from build123d import *

# Parameters (mm, degrees)
BOSS_EXTRU_1_DEPTH = 6


with BuildPart() as part:
    # Esquisse1 → Boss.-Extru.1 (new body)
    with BuildSketch(Plane.XY):
        with BuildLine():
            Line((0, 0), (6, 0))
            ThreePointArc((6, 0), (41.230424323, -8), (6, -16))
            Line((6, -16), (0, -16))
            Line((0, -16), (0, 0))
        make_face()
        with BuildLine():
            Line((3, -5), (7.5, -5))
            ThreePointArc((7.5, -5), (38.206906326, -8), (7.5, -11))
            Line((7.5, -11), (3, -11))
            Line((3, -11), (3, -5))
        make_face(mode=Mode.SUBTRACT)
    extrude(amount=BOSS_EXTRU_1_DEPTH)


solid = part.part
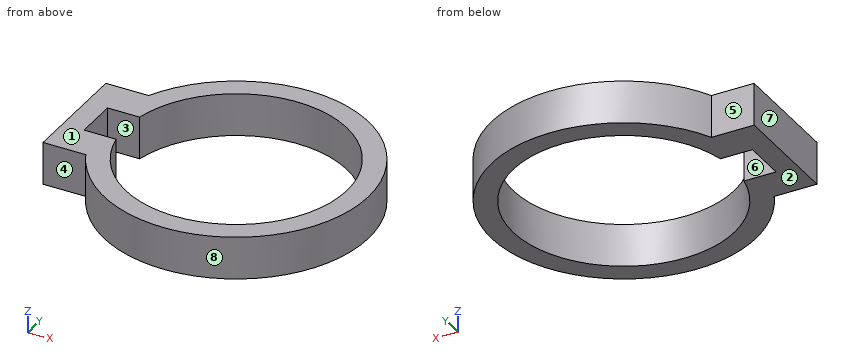
Here's how the part is built. I have some questions about the finished solid (model axes, mm). Face numbers are marked on the shaded views. A direction names the side the tool comes from. Give positions to 0.01 mm unless a question says otherwise; leave off trailing zeros. Order: outer loops, then holes, each group sorted by start corner. A loop starts at its lowest first (then second) coordinate and runs counter-clockwise, first axis right, second up. Notation, with made-up numbers: M 69.5,-30.75 L 104.5,-30.75 A16 ccw 104.5,-16.75 Z; hole C 83,-16 d7. An arc over 180 degrees is marked long. Answer as a JSON object with one key per item and string values. Group by question number.
1) Suppose I cut it at C-C, the plane z = 1.8. Write out the boundary of the cut face in (x, y), plus the area to 3 significant figures.
2) Please list where these lines run through material, in increasing order: L1, parallel to Y at x = 4.5, z = 3.05; L2, parallel to Y at x = 25.5, z = 4.35; L3, parallel to X at y = -1.5, z = 5.2. Write a range as [from, to].
3) I'm going to push flat-ended pins straight in: pin 1 Ø3 at (x, z) = (3, 4) entering from -Y; pin 2 Ø1 at (y, z) = (3, 3.5) entering from +X; pin 3 Ø1.5 at (x, z) = (32, 2.5) entering from -Y. Where does each tip first touch, or does it pass through?
4) Suppose I cut it at A-A, the plane y = -8. Write out the boundary of the cut face in (x, z), plus the area to 3 significant figures.
5) We'd pull the mould along X, two halves only. Please class the marked faces 6, 7 and 8: pulls with the +X half, pulls with the -X half, needs draft (parallel to the pull), parting line crosses it, or undercut.
6) On a 3-axis mill with a long thin cutter (end or side, diameter ignored), from which of +Z, -Z, +X, -X, +Y, -Y can I reach the whole of each face in a straight line? I mean the marked faces 1, 2, 3, 4 and 5. Say none if no direction works.
7) Suppose I cut it at B-B, the plane x = 31.5. Write out the boundary of the cut face in (y, z).
8) Suppose I cut it at D-D, the plane y = 8. Write out the boundary of the cut face in (x, z).
Results found:
{
 "1": {"outline": "M 0,-16 L 6,-16 A18.52 ccw long 6,0 L 0,0 Z; hole M 3,-11 L 7.5,-11 A15.5 ccw long 7.5,-5 L 3,-5 Z", "area": "374 mm²"},
 "2": {"L1": "[-16, -11], [-5, 0]", "L2": "[-26.31, -23.25], [7.25, 10.31]", "L3": "[0, 8.64], [36.78, 40.05]"},
 "3": {"pin 1": "y = -16", "pin 2": "x = 37.97", "pin 3": "y = -24.44"},
 "4": {"outline": "M 0,0 L 3,0 L 3,6 L 0,6 Z; M 38.21,0 L 41.23,0 L 41.23,6 L 38.21,6 Z", "area": "36.1 mm²"},
 "5": {"face 6": "undercut", "face 7": "pulls with the -X half", "face 8": "parting line crosses it"},
 "6": {"face 1": "+Z, +X, -X, +Y, -Y", "face 2": "-Z, +X, -X, +Y, -Y", "face 3": "+Z, -Z", "face 4": "+Z, -Z, -X, -Y", "face 5": "+Z, -Z, -X, +Y"},
 "7": {"outline": "M -24.3,0 L -20.76,0 L -20.76,6 L -24.3,6 Z; M 4.76,0 L 8.3,0 L 8.3,6 L 4.76,6 Z"},
 "8": {"outline": "M 13.37,0 L 32.04,0 L 32.04,6 L 13.37,6 Z"}
}
